Model file for the job. Use its own axes, mm. Face numbers are marked on the shaded views. A direction names the side the tool comes from. Round coordinates to 2 decimals unless told otherwise and drop trailing zeros. Order: outer loops, then holes, each group sorted by start corner. A loop starts at its lowest first (then second) coordinate and runs counter-clockwise, first axis right, second up. Notation, with made-up numbers: (-21.5, 10) - (17.5, 10) arc R15 cw to (17.5, 14) - close; hole circle Ø2 at (46.25, 49). An arc over 180 degrees is marked (long way). Write item = value, one per line.
```python
from build123d import *

# Parameters (mm, degrees)
SKETCH1_W                                       = 98
SKETCH1_H                                       = 26
BOSS_EXTRUDE1_DEPTH                             = 6.5
BOSS_EXTRUDE2_DEPTH                             = 2
CUT_EXTRUDE2_DEPTH                              = 3
CUT_EXTRUDE2_DEPTH_BACK                         = 7.5
BOSS_EXTRUDE3_DEPTH                             = 0.8
SKETCH6_W                                       = 3
SKETCH6_H                                       = 15
BOSS_EXTRUDE4_DEPTH                             = 2
CHAMFER1_SIZE                                   = 0.8
CSK_FOR_M3_FLAT_HEAD_MACHINE_SCREW1_D           = 3.2
CSK_FOR_M3_FLAT_HEAD_MACHINE_SCREW1_CSINK_D     = 6.3
CSK_FOR_M3_FLAT_HEAD_MACHINE_SCREW1_CSINK_ANGLE = 90
SKETCH12_R                                      = 2
CUT_EXTRUDE3_DEPTH                              = 5


with BuildPart() as part:
    # Sketch1 → Boss-Extrude1 (new body)
    with BuildSketch(Plane.XY):
        with Locations((-4.722668085, 59.458490272)):
            Rectangle(SKETCH1_W, SKETCH1_H)
    extrude(amount=BOSS_EXTRUDE1_DEPTH)

    # Sketch3 → Boss-Extrude2 (add)
    with BuildSketch(Plane(origin=(0, 0, 0), x_dir=(-1, 0, 0), z_dir=(0, 0, -1))):
        Polygon((-44.277331915, 72.458490272), (-44.277331915, 57.458490272), (-42.277331915, 57.458490272), (-42.277331915, 70.458490272), (-39.277331915, 70.458490272), (-39.277331915, 72.458490272), align=None)
    extrude(amount=BOSS_EXTRUDE2_DEPTH)

    # Sketch4 → Cut-Extrude2 (cut, two sides)
    with BuildSketch(Plane(origin=(0, 0, 0), x_dir=(-1, 0, 0), z_dir=(0, 0, -1))) as cut_extrude2_sk:
        with BuildLine():
            Line((-44.277331915, 57.458490272), (-19.277331915, 57.458490272))
            add(Edge.make_bspline(
                [(-19.277331915, 57.458490272), (-7.832942992, 57.458490272), (8.904121741, 55.154017843), (29.529578832, 46.458490272), (40.722668085, 46.458490272)],
                knots=[0, 0, 0, 0, 0.448705595, 1, 1, 1, 1], degree=3))
            Line((40.722668085, 46.458490272), (-44.277331915, 46.458490272))
            Line((-44.277331915, 46.458490272), (-44.277331915, 57.458490272))
        make_face()
        with BuildLine():
            Line((18.722668085, 72.458490272), (53.722668085, 72.458490272))
            Line((53.722668085, 72.458490272), (53.722668085, 65.458490272))
            add(Edge.make_bspline(
                [(18.722668085, 72.458490272), (24.237785364, 72.458490272), (33.045165364, 69.996464802), (44.178399876, 65.548896557), (50.961091511, 65.458490272), (53.722668085, 65.458490272)],
                knots=[0, 0, 0, 0, 0.451492406, 0.761184281, 1, 1, 1, 1], degree=3))
        make_face()
    extrude(amount=CUT_EXTRUDE2_DEPTH, mode=Mode.SUBTRACT)
    extrude(cut_extrude2_sk.sketch, amount=-CUT_EXTRUDE2_DEPTH_BACK, mode=Mode.SUBTRACT)

    # Sketch5 → Boss-Extrude3 (add)
    with BuildSketch(Plane(origin=(0, 0, 0), x_dir=(-1, 0, 0), z_dir=(0, 0, -1))):
        with BuildLine():
            Line((43.222668085, 46.458490272), (40.722668085, 46.458490272))
            Line((40.722668085, 46.458490272), (40.722668085, 64.958490272))
            Line((40.722668085, 64.958490272), (41.222668085, 65.458490272))
            Line((41.222668085, 65.458490272), (53.722668085, 65.458490272))
            Line((53.722668085, 65.458490272), (53.722668085, 62.958490272))
            Line((53.722668085, 62.958490272), (44.122668085, 62.958490272))
            ThreePointArc((44.122668085, 62.958490272), (43.486271982, 62.694886375), (43.222668085, 62.058490272))
            Line((43.222668085, 62.058490272), (43.222668085, 46.458490272))
        make_face()
    extrude(amount=BOSS_EXTRUDE3_DEPTH)

    # Sketch6 → Boss-Extrude4 (add)
    with BuildSketch(Plane(origin=(0, 0, -2), x_dir=(-1, 0, 0), z_dir=(0, 0, -1))):
        with Locations((-42.777331915, 64.958490272)):
            Rectangle(SKETCH6_W, SKETCH6_H)
    extrude(amount=BOSS_EXTRUDE4_DEPTH)

    # Chamfer1
    chamfer1_edges = [part.edges().sort_by_distance(p)[0] for p in [
        (42.277331915, 63.958490272, -2),
    ]]
    chamfer(chamfer1_edges, length=CHAMFER1_SIZE)

    # CSK for M3 Flat Head Machine Screw1 (through all)
    with Locations(Plane.XY.offset(6.5)):
        with Locations((-49.722668085, 56.458490272)):
            CounterSinkHole(CSK_FOR_M3_FLAT_HEAD_MACHINE_SCREW1_D / 2, CSK_FOR_M3_FLAT_HEAD_MACHINE_SCREW1_CSINK_D / 2, counter_sink_angle=CSK_FOR_M3_FLAT_HEAD_MACHINE_SCREW1_CSINK_ANGLE)

    # Sketch12 → Cut-Extrude3 (cut)
    with BuildSketch(Plane(origin=(0, 0, 0), x_dir=(-1, 0, 0), z_dir=(0, 0, -1))):
        with Locations((19.647668085, 68.883490272)):
            Circle(SKETCH12_R)
    extrude(amount=-CUT_EXTRUDE3_DEPTH, mode=Mode.SUBTRACT)


solid = part.part
```
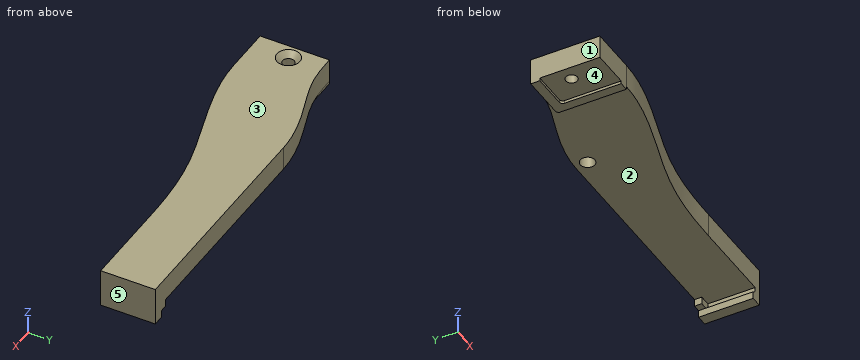
1) Cut at A-A (y = 60.5). Write the cut outline in (x, z).
Conclusion:
outline = (-53.72, 0) - (-43.22, 0) - (-43.22, -0.8) - (-40.72, -0.8) - (-40.72, 0) - (42.28, 0) - (42.28, -1.2) - (41.48, -2) - (41.28, -2) - (41.28, -4) - (44.28, -4) - (44.28, 6.5) - (-53.72, 6.5) - close
2) 3-axis set-ups, long thin cutter, end or side, ignore diameter. For the marked faces 4 and 5: which of +Z, -Z, +X, -X, +Y, -Y reach the whole face in a straight line?
Conclusion:
face_4 = -Z, -X, -Y
face_5 = +Z, -Z, +X, +Y, -Y
3) Flat gauge pins, fed straight in: pin 1 Ø4 at (x, z) = (29, -1.5) entering from -Y; pin 2 Ø2.5 at (x, y) = (-19.65, 68.88) entering from -Z; pin 3 Ø10.5 at (x, y) = (-44.5, 57) entering from -Z. Where does each tip first touch, or does it go through?
Conclusion:
pin_1 = 57.46
pin_2 = 5
pin_3 = -0.8
4) Mould opens along X. For the marked faces 1, 2 and 3 say: +X half, -X half, draft (parallel to the pull), parting line (faces both ways), or undercut.
Conclusion:
face_1 = -X half
face_2 = undercut
face_3 = draft
5) Wall check: line 1 along Z through (x, y) = (-18.5, 65.25); line 2 along X through (y, z) = (62.75, -1); line 3 along Y through (x, z) = (26, 3.75). Give the ranges that are in metal, low to high.
Conclusion:
line_1 = 0 to 6.5
line_2 = 42.28 to 44.28
line_3 = 57.46 to 72.46
6) Cut at B-B (z = 3.25). Give the number of separate pieces and of enclosed holes in the cut face, and give its area (3 significant figures).
Conclusion:
separate_pieces = 1
enclosed_holes = 2
area = 1,750 mm^2
7) Cut at C-C (x = 36). Write the cut outline in (y, z), and give its area (3 significant figures).
Conclusion:
outline = (57.46, 0) - (72.46, 0) - (72.46, 6.5) - (57.46, 6.5) - close
area = 97.5 mm^2
